Check sheet for the modelled part. Datum: model origin and axes. Units: mm. Give positions to 0.01 mm unless a question says otherwise; leave off trailing zeros. Write each loop counter-clockwise with the first axis right and the second up, starting at its lowest first coordinate (ties: lowest second). Pieces come first, ordered by that corner, then holes. Notation, with made-up numbers: (8, 39.5) -> (19, 39.5) arc R21 cw to (19, 74.5) -> close; hole circle Ø5 at (20, 80). An arc over 180 degrees is marked (long way). Return JSON: item names as keys, results as strings.
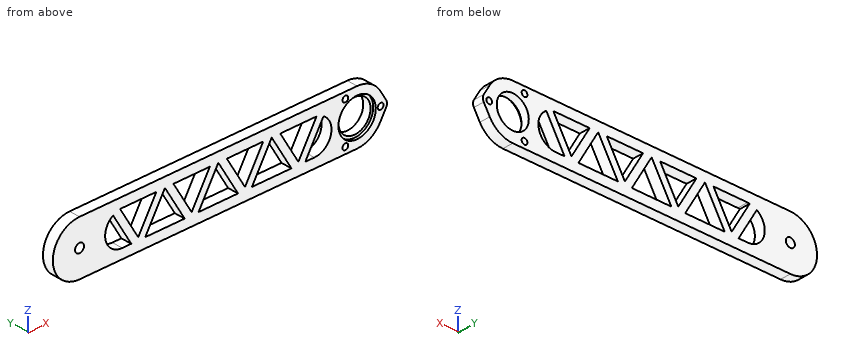
from build123d import *

# Parameters (mm, degrees)
EXTRUDE_1_DEPTH        = 5
EXTRUDE_5_DEPTH        = 5
CUT_EXTRUDE_2_REACH    = 82.139
SKETCH_7_R             = 7.5
SKETCH_8_R             = 8.75
CUT_EXTRUDE_3_DEPTH    = 1.3
CUT_EXTRUDE_4_REACH    = 82.139
SKETCH_9_R             = 1.35
CUT_EXTRUDE_5_REACH    = 82.139
SKETCH_12_R            = 2.1
CUT_EXTRUDE_6_REACH    = 82.139
EXTRUDE_6_DEPTH        = 5
PATTERN_LINEAR_1_DEPTH = 5


# Read off the part's stored shape, not the designer's step: 阵列(线性)1
with BuildPart() as part:
    # 草图1 → 凸台-拉伸1 (new body)
    with BuildSketch(Plane(origin=(0, 0, 0), x_dir=(1, 0, 0), z_dir=(0, 1, 0))):
        with BuildLine():
            Line((-65, 12.5), (65, 12.5))
            ThreePointArc((65, 12.5), (77.5, 0), (65, -12.5))
            Line((65, -12.5), (-65, -12.5))
            ThreePointArc((-65, -12.5), (-77.5, 0), (-65, 12.5))
        make_face()
    extrude(amount=EXTRUDE_1_DEPTH)

    # 草图10 → 凸台-拉伸5 (add)
    with BuildSketch(Plane.XZ):
        with BuildLine():
            Line((75.795454545, -6.301441197), (78.590909091, -1.512345887))
            ThreePointArc((78.590909091, -1.512345887), (79, 0), (78.590909091, 1.512345887))
            Line((78.590909091, 1.512345887), (75.795454545, 6.301441197))
            Line((75.795454545, 6.301441197), (75.795454545, -6.301441197))
        make_face()
    extrude(amount=-EXTRUDE_5_DEPTH)

    # 草图7 → 切除-拉伸2 (cut, up to next)
    with BuildSketch(Plane(origin=(0, 5, 0), x_dir=(1, 0, 0), z_dir=(0, 1, 0)), mode=Mode.PRIVATE) as cut_extrude_2_sk1:
        with Locations(Location((65, 0, 0), (0, 0, 270))):
            Circle(SKETCH_7_R)
    cut_extrude_2_tool1 = extrude(cut_extrude_2_sk1.sketch, amount=-CUT_EXTRUDE_2_REACH, mode=Mode.PRIVATE) & part.part
    add(cut_extrude_2_tool1.solids().sort_by_distance((65, 5, 0))[0], mode=Mode.SUBTRACT)

    # 草图8 → 切除-拉伸3 (cut)
    with BuildSketch(Plane(origin=(0, 0, 0), x_dir=(1, 0, 0), z_dir=(0, 1, 0))):
        with Locations(Location((65, 0, 0), (0, 0, 270))):
            Circle(SKETCH_8_R)
    extrude(amount=CUT_EXTRUDE_3_DEPTH, mode=Mode.SUBTRACT)

    # 草图9 → 切除-拉伸4 (cut, up to next)
    with BuildSketch(Plane.XZ, mode=Mode.PRIVATE) as cut_extrude_4_sk1:
        with Locations(Location((59.5, 9.526279442, 0), (0, 0, 270))):
            Circle(SKETCH_9_R)
    cut_extrude_4_tool1 = extrude(cut_extrude_4_sk1.sketch, amount=-CUT_EXTRUDE_4_REACH, mode=Mode.PRIVATE) & part.part
    # 草图9 → 切除-拉伸4 (cut, up to next)
    with BuildSketch(Plane.XZ, mode=Mode.PRIVATE) as cut_extrude_4_sk2:
        with Locations(Location((76, 0, 0), (0, 0, 270))):
            Circle(SKETCH_9_R)
    cut_extrude_4_tool2 = extrude(cut_extrude_4_sk2.sketch, amount=-CUT_EXTRUDE_4_REACH, mode=Mode.PRIVATE) & part.part
    # 草图9 → 切除-拉伸4 (cut, up to next)
    with BuildSketch(Plane.XZ, mode=Mode.PRIVATE) as cut_extrude_4_sk3:
        with Locations(Location((59.5, -9.526279442, 0), (0, 0, 270))):
            Circle(SKETCH_9_R)
    cut_extrude_4_tool3 = extrude(cut_extrude_4_sk3.sketch, amount=-CUT_EXTRUDE_4_REACH, mode=Mode.PRIVATE) & part.part
    add(cut_extrude_4_tool1.solids().sort_by_distance((59.5, 0, 9.526279))[0], mode=Mode.SUBTRACT)
    add(cut_extrude_4_tool2.solids().sort_by_distance((76, 0, 0))[0], mode=Mode.SUBTRACT)
    add(cut_extrude_4_tool3.solids().sort_by_distance((59.5, 0, -9.526279))[0], mode=Mode.SUBTRACT)

    # 草图12 → 切除-拉伸5 (cut, up to next)
    with BuildSketch(Plane(origin=(0, 5, 0), x_dir=(1, 0, 0), z_dir=(0, 1, 0)), mode=Mode.PRIVATE) as cut_extrude_5_sk1:
        with Locations(Location((-65, 0, 0), (0, 0, 270))):
            Circle(SKETCH_12_R)
    cut_extrude_5_tool1 = extrude(cut_extrude_5_sk1.sketch, amount=-CUT_EXTRUDE_5_REACH, mode=Mode.PRIVATE) & part.part
    add(cut_extrude_5_tool1.solids().sort_by_distance((-65, 5, 0))[0], mode=Mode.SUBTRACT)

    # 草图13 → 切除-拉伸6 (cut, up to next)
    with BuildSketch(Plane(origin=(0, 5, 0), x_dir=(1, 0, 0), z_dir=(0, 1, 0)), mode=Mode.PRIVATE) as cut_extrude_6_sk1:
        with BuildLine():
            Line((-45, 8), (45, 8))
            ThreePointArc((45, 8), (53, 0), (45, -8))
            Line((45, -8), (-45, -8))
            ThreePointArc((-45, -8), (-53, 0), (-45, 8))
        make_face()
    cut_extrude_6_tool1 = extrude(cut_extrude_6_sk1.sketch, amount=-CUT_EXTRUDE_6_REACH, mode=Mode.PRIVATE) & part.part
    add(cut_extrude_6_tool1.solids().sort_by_distance((0, 5, 0))[0], mode=Mode.SUBTRACT)

    # 草图14 → 凸台-拉伸6 (add)
    with BuildSketch(Plane(origin=(0, 5, 0), x_dir=(1, 0, 0), z_dir=(0, 1, 0))):
        Polygon((0, -8), (9.237604307, 8), (13.237604307, 8), (4, -8), align=None)
    extrude_6 = extrude(amount=-EXTRUDE_6_DEPTH)

    # 阵列(线性)1 outline → 阵列(线性)1 (add)
    with BuildSketch(Plane(origin=(0, 0, 0), x_dir=(1, 0, 0), z_dir=(0, 1, 0))):
        Polygon((38.237604307, 8), (34.237604307, 8), (25, -8), (29, -8), align=None)
        Polygon((-11.762395693, 8), (-15.762395693, 8), (-25, -8), (-21, -8), align=None)
        with BuildLine():
            Line((-45.966190603, -7.941440406), (-36.762395693, 8))
            Line((-36.762395693, 8), (-40.762395693, 8))
            Line((-40.762395693, 8), (-49.282491188, -6.757238284))
            ThreePointArc((-49.282491188, -6.757238284), (-47.690306451, -7.534072683), (-45.966190603, -7.941440406))
        make_face()
    pattern_linear_1 = extrude(amount=PATTERN_LINEAR_1_DEPTH)

    # 镜向1: 凸台-拉伸6, 阵列(线性)1 across plane
    add(extrude_6.mirror(Plane(origin=(0, 0, 0), x_dir=(0, 0, 1), z_dir=(1, 0, 0))))
    add(pattern_linear_1.mirror(Plane(origin=(0, 0, 0), x_dir=(0, 0, 1), z_dir=(1, 0, 0))))


solid = part.part
(1) Cross-section at B-B on y = 4.15. State how many separate pieces and enclosed holes the cut face has, then the cut area to 3 significant figures.
Reply:
{"separate pieces": "1", "enclosed holes": "14", "area": "2,400 mm^2"}
(2) Thickness scan on L1, parallel to Z at x = 34.5, y = 0.75; L2, parallel to X at y = 3.65, z = 8.5; L3, parallel to Y at x = 71, z = -5.5. Record the ranges inside material, lowest first.
Reply:
{"L1": "-12.5 to -1.53, 8 to 12.5", "L2": "-74.17 to 58.62, 60.38 to 74.17", "L3": "1.3 to 5"}
(3) Cross-section at A-A on x = 59.5. Enter the section's corners in (y, z), then the cut area to 3 significant figures.
Reply:
{"outline": "(0, -12.5) -> (5, -12.5) -> (5, -10.88) -> (0, -10.88) -> close; (0, -8.18) -> (5, -8.18) -> (5, -5.1) -> (1.3, -5.1) -> (1.3, -6.81) -> (0, -6.81) -> close; (0, 6.81) -> (1.3, 6.81) -> (1.3, 5.1) -> (5, 5.1) -> (5, 8.18) -> (0, 8.18) -> close; (0, 10.88) -> (5, 10.88) -> (5, 12.5) -> (0, 12.5) -> close", "area": "42.6 mm^2"}
